Geometry: see drawing. Coordinates: mm, zero at the bounding-box minimum. A direction names the side the tool comes from. Coordinates: 2 decimals unless noted, no trailing zeros. Loops run counter-clockwise (first coordinate to the right, second up) from the corner with the lowest first, then second, coordinate; pieces in that order, holes last. Notation, with made-up numbers: (83, 9) -> (115, 9) arc R23 ccw to (115, 35) -> close; hole circle Ø8 at (86.5, -39.75). An arc over 180 degrees is marked (long way). Put each result on its own line as item: value. Start each with the question number.
1) Cut plane A-A (y = 5). Return the cut outline in (x, z), plus the area to 3 significant figures.
2) Cut plane D-D (y = 18.5). Return the cut outline in (x, z).
3) Material intervals for L1, parallel to Y at x = 26, z = 3; L2, parallel to Y at x = 32.75, z = 90.05; L3, parallel to Z at x = 25.5, y = 10.5 (1 decimal), sorted ascending.
4) Cut plane B-B (x = 32.75). Return the cut outline in (y, z), plus the area to 3 significant figures.
5) Pull-direction query (Z, two-part tool) for the marked faces 1, 2 and 3; classes: pulls with the +Z half, pulls with the -Z half, needs draft (parallel to the pull), parting line crosses it, or undercut.
6) Contact query for flat-ended pins moving along their axis: P1, Ø2, axis at x = 32, y = 2.5, coming from the -Z side; P2, Ø5, axis at y = 10.5, z = 13.5, coming from the +X side; P3, Ø8, axis at x = 11.5, z = 19.5, coming from the -Y side. Output: stop coordinate, or through.
7) Cut plane C-C (y = 10). Return the cut outline in (x, z), plus the area to 3 significant figures.
8) Set-up query: the marked faces 4, 5, 6 and 7. Return all of +Z, -Z, +X, -X, +Y, -Y with unobstructed straight access to the full face (end or side cutting, diameter ignored); none if empty.
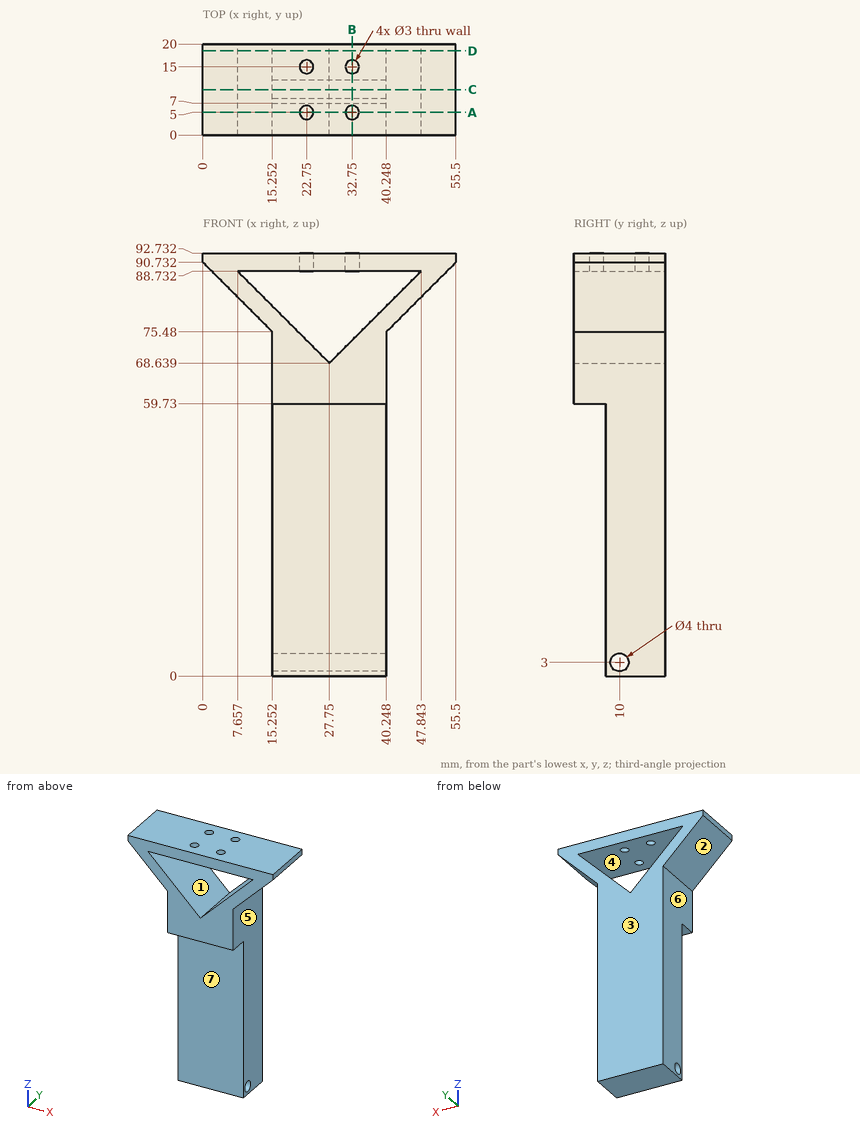
Results found:
1. outline: (0, 90.73) -> (15.25, 75.48) -> (15.25, 59.73) -> (40.25, 59.73) -> (40.25, 75.48) -> (55.5, 90.73) -> (55.5, 92.73) -> (34.25, 92.73) -> (34.25, 88.73) -> (47.84, 88.73) -> (27.75, 68.64) -> (7.66, 88.73) -> (21.25, 88.73) -> (21.25, 92.73) -> (0, 92.73) -> close; (24.25, 88.73) -> (31.25, 88.73) -> (31.25, 92.73) -> (24.25, 92.73) -> close
1. area: 691 mm2
2. outline: (0, 90.73) -> (15.25, 75.48) -> (15.25, 0) -> (40.25, 0) -> (40.25, 75.48) -> (55.5, 90.73) -> (55.5, 92.73) -> (0, 92.73) -> close; hole (7.66, 88.73) -> (27.75, 68.64) -> (47.84, 88.73) -> close
3. L1: y = 7 to 8, 12 to 20
3. L2: y = 0 to 3.5, 6.5 to 13.5, 16.5 to 20
3. L3: z = 0 to 1.1, 4.9 to 70.9, 88.7 to 92.7
4. outline: (0, 59.73) -> (7, 59.73) -> (7, 0) -> (20, 0) -> (20, 73.64) -> (0, 73.64) -> close; (0, 88.73) -> (3.5, 88.73) -> (3.5, 92.73) -> (0, 92.73) -> close; (6.5, 88.73) -> (13.5, 88.73) -> (13.5, 92.73) -> (6.5, 92.73) -> close; (16.5, 88.73) -> (20, 88.73) -> (20, 92.73) -> (16.5, 92.73) -> close; hole circle Ø4 at (10, 3)
4. area: 1,100 mm2
5. face 1: undercut
5. face 2: pulls with the -Z half
5. face 3: needs draft
6. P1: stops at z = 59.73
6. P2: stops at x = 40.25
6. P3: stops at y = 7
7. outline: (0, 90.73) -> (15.25, 75.48) -> (15.25, 5) -> (40.25, 5) -> (40.25, 75.48) -> (55.5, 90.73) -> (55.5, 92.73) -> (0, 92.73) -> close; (15.25, 0) -> (40.25, 0) -> (40.25, 1) -> (15.25, 1) -> close; hole (7.66, 88.73) -> (27.75, 68.64) -> (47.84, 88.73) -> close
7. area: 2,110 mm2
8. face 4: +Y, -Y
8. face 5: -Z, +X, +Y, -Y
8. face 6: -Z, -X, +Y, -Y
8. face 7: -Z, +X, -X, -Y
